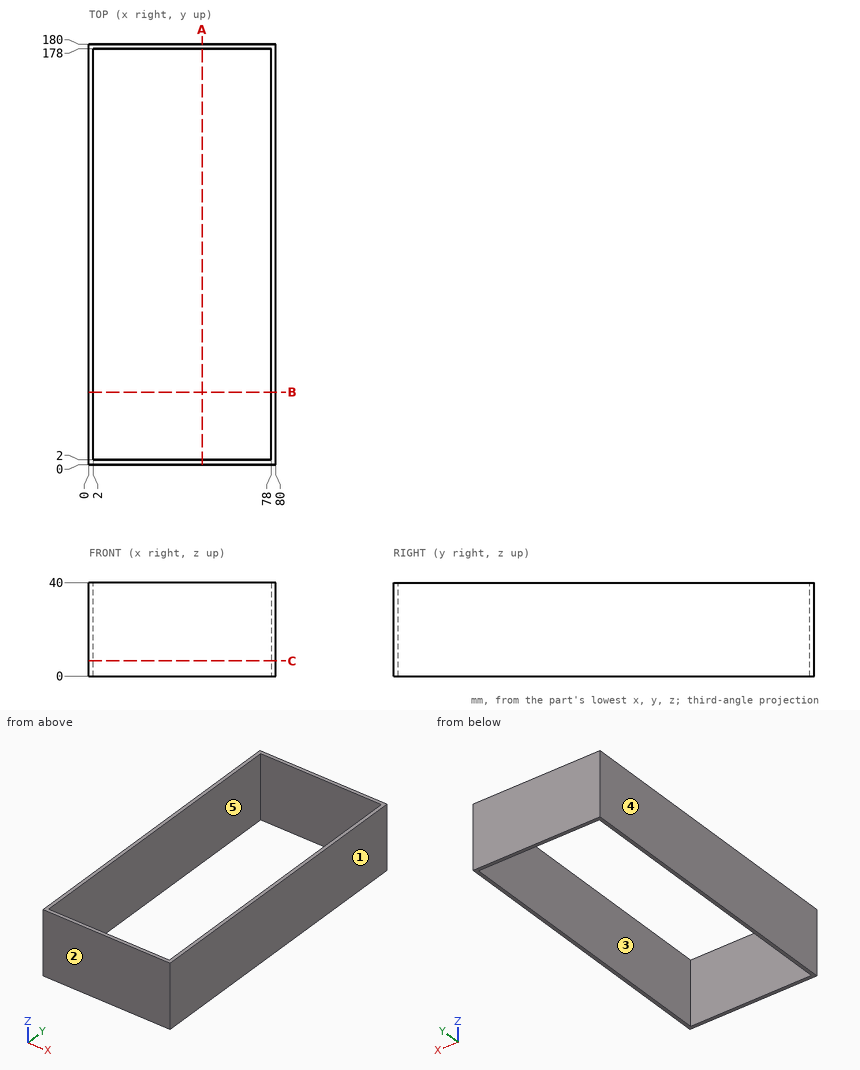
Design review of the part shown in the three views and the two pictorial views. Dimensions are in mm from the part's minimum x, y and z. A direction names the side the tool comes from. Round coordinates to 2 decimals unless told otherwise and drop trailing zeros. Write each loop counter-clockwise with the first axis right and the second up, starting at its lowest first coordinate (ties: lowest second). Pieces come first, ordered by that corner, then holes. Notation, with made-up numbers: M -15,-20 L 18,-20 A17 cw 18,7 Z; hole C 9,32 d7. An arc over 180 degrees is marked long. One line per item, written item: value. Start each with the question number.
1. For the marked faces 4 and 5, list the 3-axis set-ups (+Z, -Z, +X, -X, +Y, -Y) from which the entire face can be reached by the end or side of a thin tool; tool diameter is ignored.
2. To check wall thickness, follow probe 1 along Y at (x, z) = (16, 25); probe 2 along X at (y, z) = (131.5, 31.5). State the ranges of each line that lie inside material, in increasing order. Write a range as from..to.
3. Take a section at A-A on x = 48.5. State the section outline as (y, z) points.
4. Draft analysis for pull direction X (two halves, no side actions). For the marked faces 1, 2 and 3, state which applies: pulls with the +X half, pulls with the -X half, needs draft (parallel to the pull), parting line crosses it, or undercut.
5. Take a section at C-C on z = 6.5. State the section outline as (x, y) points, then the cut area to 3 significant figures.
6. Take a section at B-B on y = 31. State the section outline as (x, z) points, then the cut area to 3 significant figures.
Computed:
1. face 4: +Z, -Z, -X, +Y, -Y
1. face 5: +Z, -Z
2. probe 1: y = 0..2, 178..180
2. probe 2: x = 0..2, 78..80
3. outline: M 0,0 L 2,0 L 2,40 L 0,40 Z; M 178,0 L 180,0 L 180,40 L 178,40 Z
4. face 1: pulls with the +X half
4. face 2: needs draft
4. face 3: undercut
5. outline: M 0,0 L 80,0 L 80,180 L 0,180 Z; hole M 2,2 L 78,2 L 78,178 L 2,178 Z
5. area: 1,020 mm²
6. outline: M 0,0 L 2,0 L 2,40 L 0,40 Z; M 78,0 L 80,0 L 80,40 L 78,40 Z
6. area: 160 mm²
